```python
from build123d import *

# Parameters (mm, degrees)
F0_W      = 30
F0_H      = 140
F1_DEPTH  = 30
F2_R      = 13.2532741624
F3_DEPTH  = 54.4
F4_R      = 14.451224753
F5_DEPTH  = 128.1
F7_DEPTH  = 70.9
F9_DEPTH  = 175.5
F11_DEPTH = 153.2
F12_R     = 8.2133766701
F13_DEPTH = 33.1
F14_R     = 13.6361041186
F15_DEPTH = 73.6


with BuildPart() as f1:
    # F0 (on Front) → F1 (new body)
    with BuildSketch(Plane.XZ):
        Rectangle(F0_W, F0_H)
    extrude(amount=F1_DEPTH)

    # F2 (on face) → F3 (cut)
    with BuildSketch(Plane.XZ.offset(30)):
        with Locations((0, 70)):
            Circle(F2_R)
    extrude(amount=-F3_DEPTH, mode=Mode.SUBTRACT)

    # F4 (on face) → F5 (cut)
    with BuildSketch(Plane.XZ.offset(30)):
        with Locations((-15, 45.1164804399)):
            Circle(F4_R)
    extrude(amount=-F5_DEPTH, mode=Mode.SUBTRACT)

    # F6 (on face) → F7 (cut)
    with BuildSketch(Plane.XZ.offset(30)):
        with BuildLine():
            ThreePointArc((-9.9419789308, 58.6536263624), (-13.0147365818, 62.199966598), (-15, 66.4516836405))
            Line((-15, 66.4516836405), (-21.4710962027, 59.249356389))
            Line((-21.4710962027, 59.249356389), (-15, 55.8520294726))
            Line((-15, 55.8520294726), (-9.9419789308, 58.6536263624))
        make_face()
    extrude(amount=-F7_DEPTH, mode=Mode.SUBTRACT)

    # F8 (on face) → F9 (cut)
    with BuildSketch(Plane(origin=(0, 0, -70), x_dir=(1, 0, 0), z_dir=(0, 0, -1))):
        with BuildLine():
            add(Edge.make_bspline(
                [(15, 23.5094930977), (11.8512469004, 24.2984324234), (4.2834443272, 26.1945915921), (-7.8910030615, 22.2687074811), (-15, 19.9762750417)],
                knots=[0, 0, 0, 0, 0.4160723102, 1, 1, 1, 1], degree=3))
            Line((15, 23.5094930977), (15, 30))
            Line((15, 30), (-15, 30))
            Line((-15, 30), (-15, 19.9762750417))
        make_face()
        Polygon((15, 30), (15, 23.5094930977), (28.6734271795, 27.3144952953), (25.2801995763, 39.5081940436), (-18.2096641511, 41.3114763796), (-27.3144952953, 36.9629003108), (-15, 19.9762750417), (-15, 30), align=None)
    extrude(amount=-F9_DEPTH, mode=Mode.SUBTRACT)

    # F10 (on face) → F11 (cut)
    with BuildSketch(Plane(origin=(0, 0, -70), x_dir=(1, 0, 0), z_dir=(0, 0, -1))):
        with BuildLine():
            add(Edge.make_bspline(
                [(-14.9482320994, 14.5405521616), (-9.960949986, 13.377550706), (0.0492499744, 11.0432377754), (10.004603164, 14.0054335818), (15, 15.491804108)],
                knots=[0, 0, 0, 0, 0.4982200289, 1, 1, 1, 1], degree=3))
            Line((-14.9482320994, 14.5405521616), (-15, 14.4570896226))
            Line((-15, 14.4570896226), (-15, 0))
            Line((-15, 0), (15, 0))
            Line((15, 0), (15, 15.491804108))
        make_face()
        Polygon((25.2761021256, 14.4046600908), (15, 15.491804108), (15, 0), (-15, 0), (-15, 14.4570896226), (-21.6069892049, 3.8050042931), (-17.8019851446, -5.2743439193), (23.1941929335, -5.2743439193), align=None)
    extrude(amount=-F11_DEPTH, mode=Mode.SUBTRACT)

    # F12 (on Right) → F13 (cut, symmetric)
    with BuildSketch(Plane.YZ):
        with Locations((-10.8714420348, 60.336496681)):
            Circle(F12_R)
    extrude(amount=F13_DEPTH, both=True, mode=Mode.SUBTRACT)

    # F14 (on Top) → F15 (cut)
    with BuildSketch(Plane.XY):
        with Locations((0, -3.8050042931)):
            Circle(F14_R)
    extrude(amount=F15_DEPTH, mode=Mode.SUBTRACT)


solid = f1.part
```
Check sheet for the modelled part. Datum: model origin and axes. Units: mm. A direction names the side the tool comes from. Give positions to 0.01 mm unless a question says otherwise; leave off trailing zeros.
Item 1: Scan lines: L1, parallel to X at y = -21, z = 45; L2, parallel to Z at x = 4, y = -16.25; L3, parallel to X at y = -22, z = 46. Record each from-to range of solid material in increasing order.
Item 2: Gauge pin test, flat ends, axial feed: pin 1 (4 mm diameter, centred on x = -1, y = -20, fed in from +Z); pin 2 (2.5 mm diameter, centred on x = -2.5, y = -15.5, fed in from +Z); pin 3 (4 mm diameter, centred on x = 8.5, z = -49.5, fed in from +Y). Record the tip position at first contact, or that the pin passes through.
Item 3: Access from +Z, -Z, +X, -X, +Y, -Y to the whole of each face (thin tool, end or side, straight path). Record for faces 1 (the face through (0, -15, 0)), 2 (the face through (-0.83, -20.02, 42.27)).
Item 4: Draft check along X on faces 3 (the face through (1.834, -17.317, 21.159)), 4 (the face through (-12.979, -19.589, 62.145)), 5 (the face through (4.26, -20.78, 57.45)), 6 (the face through (15, -19, -1)). Enter one of: released by +X, released by -X, zero draft, split by the parting line, or undercut.
Report:
1. L1: x = -0.55 to 15
1. L2: z = -70 to 0
1. L3: x = -0.58 to 15
2. pin 1: stops at z = 57.09
2. pin 2: stops at z = 0
2. pin 3: stops at y = -13.21
3. face 1: +Z, +Y
3. face 2: -X, +Y, -Y
4. face 3: undercut
4. face 4: released by -X
4. face 5: undercut
4. face 6: released by +X
